Drawing for the job (mm, zero at the part's lowest x, y, z). A direction names the side the tool comes from. Round coordinates to 2 decimals unless told otherwise and drop trailing zeros. Loops run counter-clockwise (first coordinate to the right, second up) from the corner with the lowest first, then second, coordinate; pieces in that order, holes last. Notation, with made-up numbers: M 73,49.25 L 91,49.25 A7 cw 91,57.25 Z; hole C 63.25,-17.5 d3. An arc over 180 degrees is marked long. Put each result on its own line as item: value. Start each with the question number.
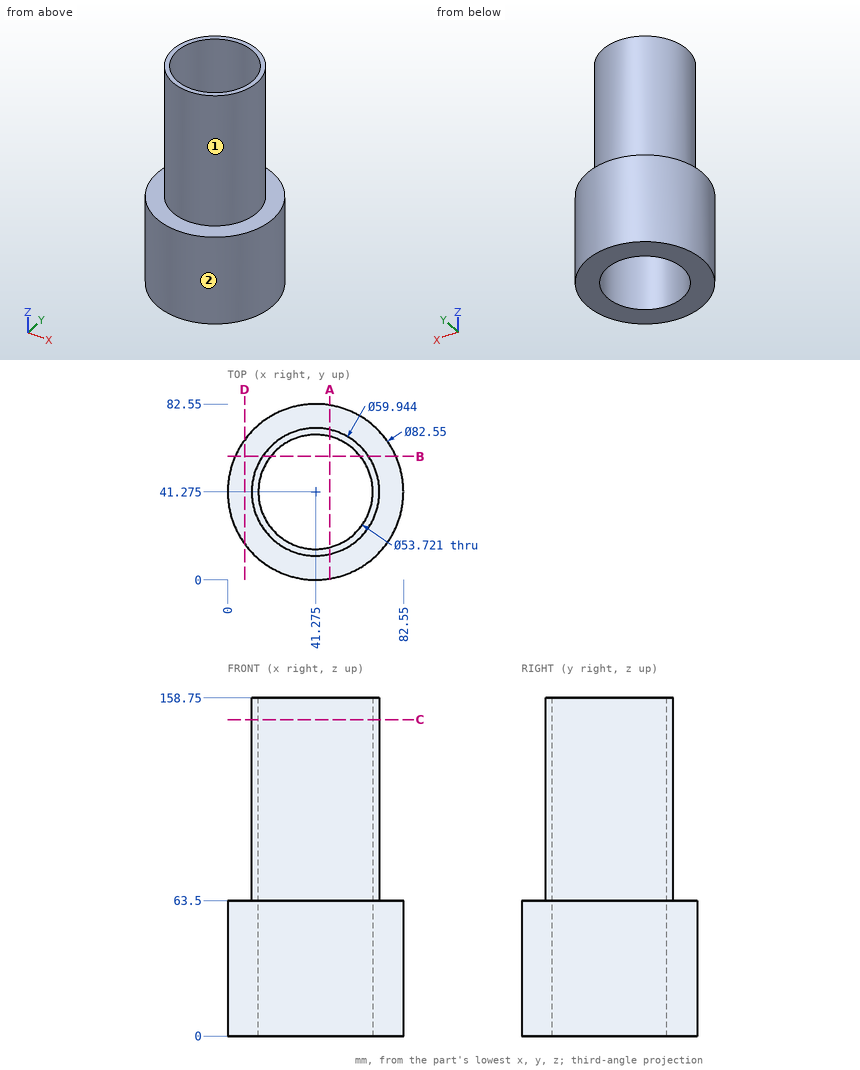
1. Which spindle directions (+Z, -Z, +X, -X, +Y, -Y) get a long thin tool onto all of the face, cutting with end or side? Do the marked faces 1 and 2. Say none if no direction does.
2. Cut at A-A, the plane x = 48. Give the cut face in (y, z).
3. Cut at D-D, the plane x = 8. Give the cut face in (y, z), and give its area (3 significant figures).
4. Drop flat-ended pins along their axis: pin 1 (3 mm diameter, centred on x = 21.5, z = 41.5, fed in from -Y); pin 2 (2 mm diameter, centred on y = 57, z = 70, fed in from +X); pin 3 (2 mm diameter, centred on x = 60, z = 110, fed in from +Y). Give the stop position or say it passes through.
5. Cut at C-C, the plane z = 148.5. Give the cut face in (x, y) (1 decimal), and give its area (3 significant figures).
6. Cut at B-B, the plane y = 58. Give the cut face in (x, z).
7. Wall check: L1, parallel to X at y = 21, z = 41; L2, parallel to Z at x = 47.5, y = 4.5; L3, parallel to X at y = 22.5, z = 66. Give the ranges that are in metal, low to high.
Results list:
1. face 1: +Z
1. face 2: +Z, -Z
2. outline: M 0.55,0 L 15.27,0 L 15.27,158.75 L 12.07,158.75 L 12.07,63.5 L 0.55,63.5 Z; M 67.28,0 L 82,0 L 82,63.5 L 70.48,63.5 L 70.48,158.75 L 67.28,158.75 Z
3. outline: M 16.85,0 L 65.7,0 L 65.7,63.5 L 16.85,63.5 Z
3. area: 3,100 mm^2
4. pin 1: stops at y = 4.27
4. pin 2: stops at x = 67.38
4. pin 3: stops at y = 65.44
5. outline: C 41.3,41.3 d59.9; hole C 41.3,41.3 d53.7
5. area: 556 mm^2
6. outline: M 3.54,0 L 20.26,0 L 20.26,158.75 L 16.4,158.75 L 16.4,63.5 L 3.54,63.5 Z; M 62.29,0 L 79.01,0 L 79.01,63.5 L 66.15,63.5 L 66.15,158.75 L 62.29,158.75 Z
7. L1: x = 5.32 to 23.66, 58.89 to 77.23
7. L2: z = 0 to 63.5
7. L3: x = 17.91 to 22.07, 60.48 to 64.64
